Autodesk Inventor part; units mm, degrees
ref_plane "YZ Plane" through (0, 0, 0) normal (1, 0, 0) x (0, 1, 0)
ref_plane "XZ Plane" through (0, 0, 0) normal (0, 1, 0) x (-1, 0, 0)
ref_plane "XY Plane" through (0, 0, 0) normal (0, 0, 1) x (1, 0, 0)
sketch "Sketch1" plane through (0, 0, 0) normal (0, 1, 0) x (-1, 0, 0)
  line L0 (0, 0) -> (-50.8, 0)
  line L1 (-50.8, 0) -> (-50.8, -25.4)
  line L2 (-50.8, -25.4) -> (0, -25.4)
  line L3 (0, -25.4) -> (0, 0)
  dimension "d0" = 50.8
  dimension "d1" = 25.4
extrude "Extrusion1" add sketch "Sketch1" along normal blind 3.175
sketch "Sketch2" plane through (0, 3.175, 0) normal (0, 1, 0) x (1, 0, 0)
  line L0 (8.89, 3.175) -> (41.91, 3.175)
  line L1 (41.91, 3.175) -> (41.91, 6.35)
  line L2 (41.91, 6.35) -> (8.89, 6.35)
  line L3 (8.89, 6.35) -> (8.89, 3.175)
  line L4 (8.89, 19.05) -> (41.91, 19.05)
  line L5 (41.91, 19.05) -> (41.91, 22.225)
  line L6 (41.91, 22.225) -> (8.89, 22.225)
  line L7 (8.89, 22.225) -> (8.89, 19.05)
  line L8 (0, 25.4) -> (0, 0)
  line L9 (50.8, 0) -> (50.8, 25.4)
  line L10 (50.8, 25.4) -> (0, 25.4)
  point P0 (41.91, 20.6375)
  point P1 (41.91, 4.7625)
  point P2 (8.89, 20.6375)
  point P3 (8.89, 4.7625)
  dimension "d4" = 8.89
  dimension "d5" = 8.89
  dimension "d6" = 3.175
  dimension "d7" = 12.7
  dimension "d8" = 3.175
extrude "Extrusion2" add sketch "Sketch2" along normal blind 38.1
sketch "Sketch3" plane through (8.89, 3.175, -3.175) normal (0, 0, 1) x (1, 0, 0)
  line L0 (0, 0) -> (0, 38.1)
  line L1 (0, 0) -> (13.8479, 21.3045)
  line L2 (19.1721, 21.3045) -> (33.02, 0)
  line L3 (33.02, 0) -> (33.02, 38.1)
  line L4 (-8.89, 0) -> (41.91, 0)
  arc A0 (19.1721, 21.3045) -> (13.8479, 21.3045) centre (16.51, 19.5742) ccw
  line L5 (33.02, 38.1) -> (0, 38.1)
  line L6 (0, 38.1) -> (33.02, 38.1)
  point P0 (-8.89, -3.175)
  point P1 (16.51, 25.4)
  dimension "d11" = 25.4
  dimension "d12" = 3.175
extrude "Extrusion3" cut sketch "Sketch3" against normal blind 38.1 contours L0 L5 L3 L2 A0 L1
sketch "Sketch4" plane through (8.89, 3.175, -3.175) normal (0, 0, 1) x (1, 0, 0)
  circle A0 centre (16.51, 12.7) radius 3.6539
  line L0 (-8.89, 0) -> (41.91, 0)
  point P0 (-8.89, -3.175)
  point P1 (16.51, 0)
  dimension "d15" = 12.7
extrude "Extrusion4" cut sketch "Sketch4" against normal blind 38.1
sketch "Sketch6" plane through (0, 3.175, 0) normal (0, 1, 0) x (1, 0, 0)
  line L0 (50.8, 0) -> (0, 0)
  line L1 (0, 0) -> (0, -3.175)
  line L2 (0, -3.175) -> (50.8, -3.175)
  line L3 (50.8, -3.175) -> (50.8, 0)
  line L4 (50.8, 28.575) -> (0, 28.575)
  line L5 (0, 28.575) -> (0, 25.4)
  line L6 (0, 25.4) -> (50.8, 25.4)
  line L7 (50.8, 25.4) -> (50.8, 28.575)
  line L8 (50.8, 0) -> (50.8, 25.4)
  line L9 (0, 25.4) -> (0, 0)
  point P0 (50.8, -1.5875)
  point P1 (50.8, 26.9875)
  point P2 (0, -1.5875)
  point P3 (0, 26.9875)
  point P4 (25.4, 0)
  point P5 (0, 12.7)
  dimension "d26" = 0
  dimension "d27" = 3.175
extrude "Extrusion5" add sketch "Sketch6" against normal blind 28.575 contours L3 L2 L1 L0 | L6 L5 L4 L7
sketch "Sketch7" plane through (0, 3.175, 3.175) normal (0, 0, 1) x (1, 0, 0)
  line L0 (0, 0) -> (50.8, 0) construction
  line L1 (0, 0) -> (0, -28.575) construction
  line L2 (50.8, -28.575) -> (0, -28.575) construction
  line L3 (50.8, 0) -> (50.8, -28.575) construction
  line L4 (44.45, -22.225) -> (6.35, -22.225) construction
  line L5 (6.35, -22.225) -> (6.35, -6.35) construction
  line L6 (6.35, -6.35) -> (44.45, -6.35) construction
  line L7 (44.45, -6.35) -> (44.45, -22.225) construction
  point P0 (0, -3.175)
  dimension "d30" = 6.35
hole "Hole2" at (6.35, -3.175, 3.175) at (44.45, -3.175, 3.175) at (44.45, -19.05, 3.175) at (6.35, -19.05, 3.175) direction (0, 0, -1) diameter 3.175 end through all
fillet "Fillet1" radius 3.175 4 edges at (0, -25.4, 1.5875) (0, -25.4, -26.9875) (50.8, -25.4, 1.5875) (50.8, -25.4, -26.9875)
ref_plane "Work Plane1" through (8.89, 3.175, -12.7) normal (0, 0, 1) x (1, 0, 0)
ref_plane "Work Plane2" through (41.91, 3.175, -3.175) normal (1, 0, 0) x (0, 0, -1)
sketch "Sketch8" plane through (41.91, 3.175, -3.175) normal (1, 0, 0) x (0, 0, -1)
  line L0 (0, 0) -> (0, 9.0461)
  line L1 (-6.35, 0) -> (-6.35, -25.4)
  line L2 (0, 9.0461) -> (-6.35, 0)
  line L3 (-6.35, 0) -> (0, 0)
  line L4 (0, 9.0461) -> (0, 16.3539)
  point P0 (-3.175, -3.175)
extrude "Extrusion6" add sketch "Sketch8" along normal blind 8.89 and the other way blind 41.91
sketch "Sketch10" plane through (14.7699, 12.2211, -3.175) normal (0, 0, -1) x (-1, 0, 0)
  line L0 (-27.1401, -9.0461) -> (-21.2601, 0)
  line L1 (-21.2601, 0) -> (-36.0301, -9.0461)
  line L2 (-36.0301, 0) -> (-36.0301, -9.0461)
  line L3 (-21.2601, 0) -> (-36.0301, 0)
  line L4 (-36.0301, -9.0461) -> (-36.0301, 0)
  line L5 (-36.0301, 0) -> (-36.0301, -9.0461)
  line L6 (0, 0) -> (5.8799, -9.0461)
  line L7 (0, 0) -> (14.7699, -9.0461)
  line L8 (14.7699, -9.0461) -> (14.7699, 0)
  line L9 (14.7699, -9.0461) -> (14.7699, 0)
  line L10 (14.7699, 0) -> (0, 0)
  point P0 (14.7699, -12.2211)
extrude "Extrusion8" cut sketch "Sketch10" against normal blind 8.89
mirror "Mirror2" about plane through (8.89, 3.175, -12.7) normal (0, 0, 1) of "Extrusion6", "Extrusion8"
sketch "Sketch11" plane through (8.89, 3.175, -3.175) normal (0, 0, -1) x (-1, 0, 0)
  line L0 (8.89, 0) -> (-5.8799, 9.0461)
  line L1 (-5.8799, 9.0461) -> (0, 0)
  line L2 (8.89, 0) -> (0, 0)
  line L3 (-27.1401, 9.0461) -> (-41.91, 0)
  line L4 (-33.02, 0) -> (-41.91, 0)
  line L5 (-33.02, 0) -> (-27.1401, 9.0461)
  point P0 (8.89, -3.175)
extrude "Extrusion9" add sketch "Sketch11" along normal blind 3.175
mirror "Mirror3" about plane through (8.89, 3.175, -12.7) normal (0, 0, 1) of "Extrusion9"
properties part number "Intake - Piston Mount"
The model under review builds one solid part; all positions refer to its coordinate system, in mm. A direction names the side the tool comes from. Round coordinates to 2 decimals unless told otherwise and drop trailing zeros. Write each loop counter-clockwise with the first axis right and the second up, starting at its lowest first coordinate (ties: lowest second). Pieces come first, ordered by that corner, then holes. Notation, with made-up numbers: (87.5, 53) - (103.5, 53) arc R33 cw to (103.5, 83) - close; hole circle Ø9 at (12, 46). An arc over 180 degrees is marked (long way). One line per item, written item: value. Start each with the question number.
1. To check wall thickness, follow L1, parallel to X at y = -19.05, z = 2.3; L2, parallel to Z at x = 28.5, y = 23 (3 decimals); L3, parallel to Z at x = 36.5, y = -14 (3 decimals). State the ranges of each line that lie inside material, in increasing order. Write a range as from..to.
2. Clearance check with flat-ended pins moving along their axes: P1, Ø1.5, axis at y = 10, z = -8.5, coming from the -X side; P2, Ø15, axis at x = 25, y = 20.5, coming from the +Z side (3 decimals); P3, Ø2, axis at x = 36.5, z = -6, coming from the -Y side; P4, Ø6, axis at y = -13.5, z = -22.5, coming from the -X side. State where each tip first meets the part, or that it passes through.
3. Consider section A-A on y = -10. Write out the cut boundary in (x, z) (3 decimals), and give its area (3 significant figures).
4. The part is to be moulded in two halves that separate along Y. For faces 4 (the face through (26, 0, -13)), 5 (the face through (18.698, 18.264, -20.615)), 6 (the face through (27.086, 12.633, -20.615)), say which applies: released by +Y, released by -Y, zero draft, split by the parting line, or undercut.
5. Consider section B-B on x = 6.35. State how many separate pieces and enclosed holes the cut face has, and give its area (3 significant figures).
6. Machinability: for faces 1 (the face through (28, 19, -3.175)), 2 (the face through (5.85, 6.76, -2.71)), 3 (the face through (26, 10, -6.35)), which of the approach directions +Z, -Z, +X, -X, +Y, -Y give a long, thin tool a straight path to every point of the face, cutting with its end or side? Answer none if there is none.
7. Consider section D-D on z = -21.5. Write out the cut boundary in (x, y) (1 decimal).
8. Consider section C-C on y = -19.05. Write out the cut boundary in (x, z) (1 decimal), and give its area (3 significant figures).
Checks:
1. L1: x = 0..4.76, 7.94..42.86, 46.04..50.8
1. L2: z = -22.225..-19.05, -6.35..-3.175
1. L3: z = -28.575..-25.4, 0..3.175
2. P1: passes through
2. P2: stops at z = -3.175
2. P3: stops at y = 0
2. P4: stops at x = 0
3. outline: (0, -28.575) - (50.8, -28.575) - (50.8, -25.4) - (0, -25.4) - close; (0, 0) - (50.8, 0) - (50.8, 3.175) - (0, 3.175) - close
3. area: 323 mm^2
4. face 4: released by -Y
4. face 5: released by +Y
4. face 6: undercut
5. separate pieces: 5
5. enclosed holes: 0
5. area: 285 mm^2
6. face 1: +Z, +X, -X, +Y
6. face 2: +Z, -Z, -X, +Y
6. face 3: +X, -X, +Y
7. outline: (0, 0) - (50.8, 0) - (50.8, 3.2) - (36, 12.2) - (28.1, 24.5) arc R3.2 ccw to (22.7, 24.5) - (14.8, 12.2) - (0, 3.2) - close; hole circle Ø7.3 at (25.4, 15.9)
8. outline: (0, -28.6) - (4.8, -28.6) - (4.8, -25.4) - (0, -25.4) - close; (0, 0) - (4.8, 0) - (4.8, 3.2) - (0, 3.2) - close; (7.9, -28.6) - (42.9, -28.6) - (42.9, -25.4) - (7.9, -25.4) - close; (7.9, 0) - (42.9, 0) - (42.9, 3.2) - (7.9, 3.2) - close; (46, -28.6) - (50.8, -28.6) - (50.8, -25.4) - (46, -25.4) - close; (46, 0) - (50.8, 0) - (50.8, 3.2) - (46, 3.2) - close
8. area: 282 mm^2
